from build123d import *

# Parameters (mm, degrees)
SKETCH1_W           = 80
SKETCH1_H           = 30
SKETCH1_W_2         = 50
BOSS_EXTRUDE1_DEPTH = 3
FILLET1_SIZE        = 60
SKETCH6_W           = 80
SKETCH6_H           = 30
CUT_EXTRUDE1_DEPTH  = 10
FILLET3_R           = 20
SKETCH8_R           = 1.55
SKETCH8_R_2         = 11.43
SKETCH8_R_3         = 1.5875
SKETCH8_R_4         = 1.5
SKETCH8_W           = 7
SKETCH8_H           = 1.5
SKETCH8_W_2         = 1.5
SKETCH8_H_2         = 7
CUT_EXTRUDE2_DEPTH  = 3
CUT_EXTRUDE3_REACH  = 256.576
SKETCH9_R           = 1.55
SKETCH9_R_2         = 0.5
SKETCH9_W           = 0.24
SKETCH9_H           = 0.24
SKETCH9_W_2         = 0.635
SKETCH9_H_2         = 0.635


with BuildPart() as part:
    # Sketch1 → Boss-Extrude1 (new body)
    with BuildSketch(Plane(origin=(0, 0, 0), x_dir=(1, 0, 0), z_dir=(0, 1, 0))):
        with Locations((-90, -15)):
            Rectangle(SKETCH1_W, SKETCH1_H)
        Polygon((0, 180), (-180, 180), (-180, 30), (-130, 30), (-50, 30), (0, 30), align=None)
        with Locations((-25, 15)):
            Rectangle(SKETCH1_W_2, SKETCH1_H)
        with Locations((-155, 15)):
            Rectangle(SKETCH1_W_2, SKETCH1_H)
        with Locations((-90, 15)):
            Rectangle(SKETCH1_W, SKETCH1_H)
    extrude(amount=BOSS_EXTRUDE1_DEPTH)

    # Fillet1
    # a fillet whose section is not a circle: 60 mm, written as the material it takes off along each edge
    with BuildSketch(Plane(origin=(0, -150, -180), x_dir=(0, 0, 1), z_dir=(0, 1, 0)), Plane(origin=(-180, -150, -180), x_dir=(1, 0, 0), z_dir=(0, 1, 0))) as fillet1_piece_1:
        with BuildLine():
            Bezier((FILLET1_SIZE, 0), (0, 0), (0, -FILLET1_SIZE), weights=[1, 0.25, 1])
            Line((0, -FILLET1_SIZE), (0, 0))
            Line((0, 0), (FILLET1_SIZE, 0))
        make_face()
    extrude(amount=303, mode=Mode.SUBTRACT)

    # Sketch6 → Cut-Extrude1 (cut)
    with BuildSketch(Plane(origin=(0, 3, 0), x_dir=(1, 0, 0), z_dir=(0, 1, 0))):
        with Locations((-90, -15)):
            Rectangle(SKETCH6_W, SKETCH6_H)
        Polygon((-180, 100), (-180, 0), (-162, 30.1112758), (-162, 67.7112758), align=None)
        Polygon((-18, 30.1112758), (0, 0), (0, 100), (-18, 67.7112758), align=None)
    extrude(amount=-CUT_EXTRUDE1_DEPTH, mode=Mode.SUBTRACT)

    # Fillet2
    # a fillet whose section is not a circle: 10 mm, written as the material it takes off along each edge
    with BuildSketch(Plane(origin=(-180, -44.070846291, 0), x_dir=(1, 0, 0), z_dir=(0, 1, 0)), Plane(origin=(0, -44.070846291, 0), x_dir=(-0.513095679808488, 0, -0.8583314181374613), z_dir=(0, 1, 0))) as fillet2_piece_1:
        with BuildLine():
            Bezier((17.628338516, 0), (0, 0), (9.045024335, 15.130956798), weights=[1, 0.333333333, 1])
            Line((9.045024335, 15.130956798), (0, 0))
            Line((0, 0), (17.628338516, 0))
        make_face()
    extrude(amount=91.141692581, mode=Mode.SUBTRACT)

    # Fillet3
    fillet3_edges = [part.edges().sort_by_distance(p)[0] for p in [
        (0, 1.5, -100),
        (-180, 1.5, -100),
    ]]
    fillet(fillet3_edges, radius=FILLET3_R)

    # Sketch8 → Cut-Extrude2 (cut)
    with BuildSketch(Plane(origin=(0, 3, 0), x_dir=(1, 0, 0), z_dir=(0, 1, 0))):
        with Locations(Location((-105.104964584, 175.33109831, 0), (0, 0, 270))):
            Circle(SKETCH8_R)
        with Locations(Location((-74.900170028, 159.13122779, 0), (0, 0, 270))):
            Circle(SKETCH8_R)
        with Locations(Location((-141.5, 141.43, 0), (0, 0, 270))):
            Circle(SKETCH8_R_2)
        with Locations(Location((-38.5, 141.43, 0), (0, 0, 270))):
            Circle(SKETCH8_R_2)
        with Locations(Location((-112, 125.592, 0), (0, 0, 270))):
            Circle(SKETCH8_R)
        with Locations(Location((-164, 125.592, 0), (0, 0, 270))):
            Circle(SKETCH8_R)
        with Locations(Location((-112, 71.592, 0), (0, 0, 270))):
            Circle(SKETCH8_R)
        with Locations(Location((-146.4125, 64.417, 0), (0, 0, 270))):
            Circle(SKETCH8_R_3)
        with Locations(Location((-133.7125, 64.417, 0), (0, 0, 270))):
            Circle(SKETCH8_R_3)
        with Locations(Location((-121.0125, 64.417, 0), (0, 0, 270))):
            Circle(SKETCH8_R_3)
        with Locations(Location((-146.4125, 33.175, 0), (0, 0, 270))):
            Circle(SKETCH8_R_3)
        with Locations(Location((-133.7125, 33.175, 0), (0, 0, 270))):
            Circle(SKETCH8_R_3)
        with Locations(Location((-121.0125, 33.175, 0), (0, 0, 270))):
            Circle(SKETCH8_R_3)
        with Locations(Location((-58.9875, 64.417, 0), (0, 0, 270))):
            Circle(SKETCH8_R_3)
        with Locations(Location((-46.2875, 64.417, 0), (0, 0, 270))):
            Circle(SKETCH8_R_3)
        with Locations(Location((-33.5875, 64.417, 0), (0, 0, 270))):
            Circle(SKETCH8_R_3)
        with Locations(Location((-33.5875, 33.175, 0), (0, 0, 270))):
            Circle(SKETCH8_R_3)
        with Locations(Location((-46.2875, 33.175, 0), (0, 0, 270))):
            Circle(SKETCH8_R_3)
        with Locations(Location((-58.9875, 33.175, 0), (0, 0, 270))):
            Circle(SKETCH8_R_3)
        with Locations(Location((-63.9, 25.5, 0), (0, 0, 270))):
            Circle(SKETCH8_R)
        with Locations(Location((-28.6, 6.5, 0), (0, 0, 270))):
            Circle(SKETCH8_R)
        with Locations(Location((-116.8, 6.5, 0), (0, 0, 270))):
            Circle(SKETCH8_R)
        with Locations(Location((-152.1, 25.5, 0), (0, 0, 270))):
            Circle(SKETCH8_R)
        with Locations(Location((-27.14, 119.392, 0), (0, 0, 270))):
            Circle(SKETCH8_R_4)
        with Locations(Location((-25.87, 71.132, 0), (0, 0, 270))):
            Circle(SKETCH8_R_4)
        with Locations((-59.5, 167.75)):
            Rectangle(SKETCH8_W, SKETCH8_H)
        with Locations((-120.5, 167.75)):
            Rectangle(SKETCH8_W, SKETCH8_H)
        with Locations((-164.25, 135.5)):
            Rectangle(SKETCH8_W_2, SKETCH8_H_2)
        with Locations((-15.75, 135.5)):
            Rectangle(SKETCH8_W_2, SKETCH8_H_2)
    extrude(amount=-CUT_EXTRUDE2_DEPTH, mode=Mode.SUBTRACT)

    # Sketch9 → Cut-Extrude3 (cut, up to next)
    with BuildSketch(Plane.XZ, mode=Mode.PRIVATE) as cut_extrude3_sk1:
        with Locations(Location((-163.2, -97, 0), (0, 0, 270))):
            Circle(SKETCH9_R)
    cut_extrude3_tool1 = extrude(cut_extrude3_sk1.sketch, amount=-CUT_EXTRUDE3_REACH, mode=Mode.PRIVATE) & part.part
    # Sketch9 → Cut-Extrude3 (cut, up to next)
    with BuildSketch(Plane.XZ, mode=Mode.PRIVATE) as cut_extrude3_sk2:
        with Locations(Location((-158.3, -135.2, 0), (0, 0, 270))):
            Circle(SKETCH9_R)
    cut_extrude3_tool2 = extrude(cut_extrude3_sk2.sketch, amount=-CUT_EXTRUDE3_REACH, mode=Mode.PRIVATE) & part.part
    # Sketch9 → Cut-Extrude3 (cut, up to next)
    with BuildSketch(Plane.XZ, mode=Mode.PRIVATE) as cut_extrude3_sk3:
        with Locations(Location((-126.25, -158, 0), (0, 0, 270))):
            Circle(SKETCH9_R)
    cut_extrude3_tool3 = extrude(cut_extrude3_sk3.sketch, amount=-CUT_EXTRUDE3_REACH, mode=Mode.PRIVATE) & part.part
    # Sketch9 → Cut-Extrude3 (cut, up to next)
    with BuildSketch(Plane.XZ, mode=Mode.PRIVATE) as cut_extrude3_sk4:
        with Locations(Location((-53.75, -158, 0), (0, 0, 270))):
            Circle(SKETCH9_R)
    cut_extrude3_tool4 = extrude(cut_extrude3_sk4.sketch, amount=-CUT_EXTRUDE3_REACH, mode=Mode.PRIVATE) & part.part
    # Sketch9 → Cut-Extrude3 (cut, up to next)
    with BuildSketch(Plane.XZ, mode=Mode.PRIVATE) as cut_extrude3_sk5:
        with Locations(Location((-21.7, -135.2, 0), (0, 0, 270))):
            Circle(SKETCH9_R)
    cut_extrude3_tool5 = extrude(cut_extrude3_sk5.sketch, amount=-CUT_EXTRUDE3_REACH, mode=Mode.PRIVATE) & part.part
    # Sketch9 → Cut-Extrude3 (cut, up to next)
    with BuildSketch(Plane.XZ, mode=Mode.PRIVATE) as cut_extrude3_sk6:
        with Locations(Location((-16.8, -97, 0), (0, 0, 270))):
            Circle(SKETCH9_R)
    cut_extrude3_tool6 = extrude(cut_extrude3_sk6.sketch, amount=-CUT_EXTRUDE3_REACH, mode=Mode.PRIVATE) & part.part
    # Sketch9 → Cut-Extrude3 (cut, up to next)
    with BuildSketch(Plane.XZ, mode=Mode.PRIVATE) as cut_extrude3_sk7:
        with Locations(Location((-76.405, -124.775, 0), (0, 0, 270))):
            Circle(SKETCH9_R_2)
    cut_extrude3_tool7 = extrude(cut_extrude3_sk7.sketch, amount=-CUT_EXTRUDE3_REACH, mode=Mode.PRIVATE) & part.part
    # Sketch9 → Cut-Extrude3 (cut, up to next)
    with BuildSketch(Plane.XZ, mode=Mode.PRIVATE) as cut_extrude3_sk8:
        with Locations(Location((-103.71, -145.095, 0), (0, 0, 270))):
            Circle(SKETCH9_R_2)
    cut_extrude3_tool8 = extrude(cut_extrude3_sk8.sketch, amount=-CUT_EXTRUDE3_REACH, mode=Mode.PRIVATE) & part.part
    # Sketch9 → Cut-Extrude3 (cut, up to next)
    with BuildSketch(Plane.XZ, mode=Mode.PRIVATE) as cut_extrude3_sk9:
        with Locations(Location((-76.405, -145.095, 0), (0, 0, 270))):
            Circle(SKETCH9_R_2)
    cut_extrude3_tool9 = extrude(cut_extrude3_sk9.sketch, amount=-CUT_EXTRUDE3_REACH, mode=Mode.PRIVATE) & part.part
    # Sketch9 → Cut-Extrude3 (cut, up to next)
    with BuildSketch(Plane.XZ, mode=Mode.PRIVATE) as cut_extrude3_sk10:
        with Locations(Location((-103.71, -124.775, 0), (0, 0, 270))):
            Circle(SKETCH9_R_2)
    cut_extrude3_tool10 = extrude(cut_extrude3_sk10.sketch, amount=-CUT_EXTRUDE3_REACH, mode=Mode.PRIVATE) & part.part
    # Sketch9 → Cut-Extrude3 (cut, up to next)
    with BuildSketch(Plane.XZ, mode=Mode.PRIVATE) as cut_extrude3_sk11:
        with Locations((-68.3, -150.77)):
            Rectangle(SKETCH9_W, SKETCH9_H)
    cut_extrude3_tool11 = extrude(cut_extrude3_sk11.sketch, amount=-CUT_EXTRUDE3_REACH, mode=Mode.PRIVATE) & part.part
    # Sketch9 → Cut-Extrude3 (cut, up to next)
    with BuildSketch(Plane.XZ, mode=Mode.PRIVATE) as cut_extrude3_sk12:
        with Locations((-111.48, -150.77)):
            Rectangle(SKETCH9_W, SKETCH9_H)
    cut_extrude3_tool12 = extrude(cut_extrude3_sk12.sketch, amount=-CUT_EXTRUDE3_REACH, mode=Mode.PRIVATE) & part.part
    # Sketch9 → Cut-Extrude3 (cut, up to next)
    with BuildSketch(Plane.XZ, mode=Mode.PRIVATE) as cut_extrude3_sk13:
        with Locations((-76.3275, -138.745)):
            Rectangle(SKETCH9_W_2, SKETCH9_H_2)
    cut_extrude3_tool13 = extrude(cut_extrude3_sk13.sketch, amount=-CUT_EXTRUDE3_REACH, mode=Mode.PRIVATE) & part.part
    # Sketch9 → Cut-Extrude3 (cut, up to next)
    with BuildSketch(Plane.XZ, mode=Mode.PRIVATE) as cut_extrude3_sk14:
        with Locations((-76.3275, -131.125)):
            Rectangle(SKETCH9_W_2, SKETCH9_H_2)
    cut_extrude3_tool14 = extrude(cut_extrude3_sk14.sketch, amount=-CUT_EXTRUDE3_REACH, mode=Mode.PRIVATE) & part.part
    # Sketch9 → Cut-Extrude3 (cut, up to next)
    with BuildSketch(Plane.XZ, mode=Mode.PRIVATE) as cut_extrude3_sk15:
        with Locations((-103.7875, -138.745)):
            Rectangle(SKETCH9_W_2, SKETCH9_H_2)
    cut_extrude3_tool15 = extrude(cut_extrude3_sk15.sketch, amount=-CUT_EXTRUDE3_REACH, mode=Mode.PRIVATE) & part.part
    # Sketch9 → Cut-Extrude3 (cut, up to next)
    with BuildSketch(Plane.XZ, mode=Mode.PRIVATE) as cut_extrude3_sk16:
        with Locations((-103.7875, -131.125)):
            Rectangle(SKETCH9_W_2, SKETCH9_H_2)
    cut_extrude3_tool16 = extrude(cut_extrude3_sk16.sketch, amount=-CUT_EXTRUDE3_REACH, mode=Mode.PRIVATE) & part.part
    add(cut_extrude3_tool1.solids().sort_by_distance((-163.2, 0, -97))[0], mode=Mode.SUBTRACT)
    add(cut_extrude3_tool2.solids().sort_by_distance((-158.3, 0, -135.2))[0], mode=Mode.SUBTRACT)
    add(cut_extrude3_tool3.solids().sort_by_distance((-126.25, 0, -158))[0], mode=Mode.SUBTRACT)
    add(cut_extrude3_tool4.solids().sort_by_distance((-53.75, 0, -158))[0], mode=Mode.SUBTRACT)
    add(cut_extrude3_tool5.solids().sort_by_distance((-21.7, 0, -135.2))[0], mode=Mode.SUBTRACT)
    add(cut_extrude3_tool6.solids().sort_by_distance((-16.8, 0, -97))[0], mode=Mode.SUBTRACT)
    add(cut_extrude3_tool7.solids().sort_by_distance((-76.405, 0, -124.775))[0], mode=Mode.SUBTRACT)
    add(cut_extrude3_tool8.solids().sort_by_distance((-103.71, 0, -145.095))[0], mode=Mode.SUBTRACT)
    add(cut_extrude3_tool9.solids().sort_by_distance((-76.405, 0, -145.095))[0], mode=Mode.SUBTRACT)
    add(cut_extrude3_tool10.solids().sort_by_distance((-103.71, 0, -124.775))[0], mode=Mode.SUBTRACT)
    add(cut_extrude3_tool11.solids().sort_by_distance((-68.3, 0, -150.77))[0], mode=Mode.SUBTRACT)
    add(cut_extrude3_tool12.solids().sort_by_distance((-111.48, 0, -150.77))[0], mode=Mode.SUBTRACT)
    add(cut_extrude3_tool13.solids().sort_by_distance((-76.3275, 0, -138.745))[0], mode=Mode.SUBTRACT)
    add(cut_extrude3_tool14.solids().sort_by_distance((-76.3275, 0, -131.125))[0], mode=Mode.SUBTRACT)
    add(cut_extrude3_tool15.solids().sort_by_distance((-103.7875, 0, -138.745))[0], mode=Mode.SUBTRACT)
    add(cut_extrude3_tool16.solids().sort_by_distance((-103.7875, 0, -131.125))[0], mode=Mode.SUBTRACT)


solid = part.part
For this review, take the finished solid that the model builds, in its own axes (mm). A direction names the side the tool comes from. Round coordinates to 2 decimals unless told otherwise and drop trailing zeros. Write item = value, one per line. Start each with the question number.
1) Insertion check: pin 1 (1 mm diameter, centred on x = -142.5, y = 1, fed in from -Z); pin 2 (1 mm diameter, centred on x = -132.5, z = -138.5, fed in from -Y); pin 3 (1.5 mm diameter, centred on y = 2.5, z = -159.5, fed in from -X); pin 4 (1 mm diameter, centred on y = 2, z = -73.5, fed in from -X). Each pin has a flat end and moves straight along its axis. Give the tip position at first contact, or say it passes through.
2) Take a section at A-A on y = 2.25. Count the separate pieces of the cut face and the enclosed holes in it, plus the area to 3 significant figures.
3) Tool access review of faces 1 (the face through (-13.585, 1.521, -22.726)), 2 (the face through (-91, 3, -91)), 3 (the face through (-169.626, 1.521, -81.391)): name each direction out of +Z, -Z, +X, -X, +Y, -Y from which nothing blocks a thin tool from reaching the whole face with its end or side.
4) To check wall thickness, follow line 1 (Z direction, x = -112, y = 1.3); line 2 (X direction, y = 1.05, z = -6.5); line 3 (X direction, y = 1.6, z = -145.5). State the ranges of each line that lie inside material, in increasing order. Write a range as from..to.
5) The part is to be moulded in two halves that separate along Z. For faces 4 (the face through (-45.455, 1.521, -150.5)), 5 (the face through (-91, 0, -91)), 6 (the face through (-10.157, 1.521, -81.78)), say which applies: +Z half, -Z half, draft (parallel to the pull), parting line (faces both ways), or undercut.
Verdict:
q1.pin_1 = -168.47
q1.pin_2 = through
q1.pin_3 = -153.19
q1.pin_4 = -165.51
q2.separate_pieces = 1
q2.enclosed_holes = 45
q2.area = 26,100 mm2
q3.face_1 = +X, +Y, -Y
q3.face_2 = +Z, -Z, +X, -X, +Y
q3.face_3 = -X, +Y, -Y
q4.line_1 = -180..-127.14, -124.04..-73.14, -70.04..0
q4.line_2 = -170.43..-118.35, -115.25..-30.15, -27.05..-9.57
q4.line_3 = -165.63..-152.18, -130.82..-104, -103.42..-76.7, -76.11..-49.18, -27.82..-14.37
q5.face_4 = undercut
q5.face_5 = draft
q5.face_6 = undercut
